Could you check a few things on this model? Use its own coordinates, in mm. Give positions to 0.01 mm unless a question says otherwise; leave off trailing zeros. Write each loop counter-clockwise with the first axis right and the second up, starting at its lowest first coordinate (ties: lowest second). Pieces come first, ordered by that corner, then holes. Notation, with made-up numbers: (23.5, 76.5) - (29.5, 76.5) arc R18 ccw to (29.5, 80.5) - close; hole circle Ø8 at (0, 81.5). An arc over 180 degrees is marked (long way). Write item = value, one per line.
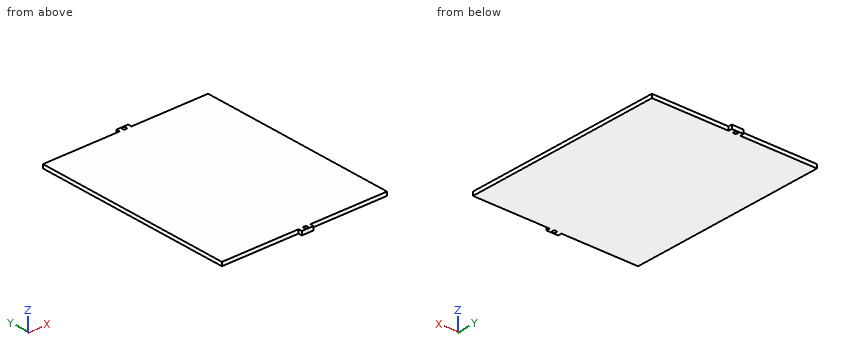
from build123d import *

# Parameters (mm, degrees)
SKETCH1_W           = 139.7
SKETCH1_H           = 177.8
BOSS_EXTRUDE1_DEPTH = 3.18
SKETCH3_R           = 1.59
SKETCH3_W           = 64.85
SKETCH3_H           = 3.18
CUT_EXTRUDE2_DEPTH  = 10


with BuildPart() as part:
    # Sketch1 → Boss-Extrude1 (new body)
    with BuildSketch(Plane.XY):
        Rectangle(SKETCH1_W, SKETCH1_H)
    extrude(amount=BOSS_EXTRUDE1_DEPTH)

    # Sketch3 → Cut-Extrude2 (cut)
    with BuildSketch(Plane.XY.offset(3.18)):
        with Locations((0, -86.9)):
            Circle(SKETCH3_R)
        with Locations((0, 86.9)):
            Circle(SKETCH3_R)
        with Locations((-37.425, -87.31)):
            Rectangle(SKETCH3_W, SKETCH3_H)
        with Locations((37.425, -87.31)):
            Rectangle(SKETCH3_W, SKETCH3_H)
        with Locations((-37.425, 87.31)):
            Rectangle(SKETCH3_W, SKETCH3_H)
        with Locations((37.425, 87.31)):
            Rectangle(SKETCH3_W, SKETCH3_H)
    extrude(amount=-CUT_EXTRUDE2_DEPTH, mode=Mode.SUBTRACT)


solid = part.part
1. If we section it at A-A, the plane z = 2.1: Please give me the cut outline in (x, y).
Filled sheet:
outline = (-69.85, -85.72) - (-5, -85.72) - (-5, -88.9) - (5, -88.9) - (5, -85.72) - (69.85, -85.72) - (69.85, 85.72) - (5, 85.72) - (5, 88.9) - (-5, 88.9) - (-5, 85.72) - (-69.85, 85.72) - close; hole circle Ø3.18 at (0, -86.9); hole circle Ø3.18 at (0, 86.9)
2. For pin 1 (3 mm diameter, centred on x = 0, y = 86.9, fed in from +Z); pin 2 (1 mm diameter, centred on x = -24, z = 2, fed in from -Y); pin 3 (1 mm diameter, centred on y = 88, z = 1, fed in from +X); pin 4 (1 mm diameter, centred on x = 46.5, z = 1.5, fed in from +Y), each with a flat end and sliding along its axis, tell me the tip position at first contact or that it passes through.
Filled sheet:
pin_1 = through
pin_2 = -85.72
pin_3 = 5
pin_4 = 85.72
3. I need wall thicknesses on line 1 (Y direction, x = 0, z = 2.15); line 2 (X direction, y = 86.9, z = 1.95); line 3 (Y direction, x = -34, z = 2.95). Which ranges of each line are inside material? Lowest first, please.
Filled sheet:
line_1 = -88.9 to -88.49, -85.31 to 85.31, 88.49 to 88.9
line_2 = -5 to -1.59, 1.59 to 5
line_3 = -85.72 to 85.72
